The model under review builds one solid part; all positions refer to its coordinate system, in mm. Give positions to 0.01 mm unless a question says otherwise; leave off trailing zeros. Loops run counter-clockwise (first coordinate to the right, second up) from the corner with the lowest first, then second, coordinate; pieces in that order, holes last. Notation, with made-up numbers: (-29, 38) -> (-8, 38) arc R27 cw to (-8, 65) -> close; hole circle Ø11 at (49.5, 43). An arc over 180 degrees is marked (long way). Write each question's results on one line, items separated by ' | '. Start each with the question number.
Q1. We need section A-A (y = 0). Write out the cut boundary in (x, z) (3 decimals).
Q2. We need section B-B (x = 27). Write out the cut boundary in (y, z), plus the area to 3 significant figures.
Q3. Wall thickness on L1, parallel to X at y = 0, z = 0.45; L2, parallel to Y at x = 11.5, z = 0; L3, parallel to Y at x = 12.5, z = 0.8: over which ranges is each line inside the solid? List them lowest first. Write a range as [from, to].
Q4. Insertion check: pin 1 Ø1.4 at (x, y) = (26, 0) entering from -Z; pin 2 Ø2 at (y, z) = (-1.5, -1.5) entering from +X; pin 3 Ø1.5 at (x, z) = (13, 0.5) entering from +Y; pin 4 Ø3 at (y, z) = (0, 1) entering from -X. Each pin has a flat end and moves straight along its axis. Give the tip position at first contact, or say it passes through.
Q5. We need section C-C (x = 14.25). Write out the cut boundary in (y, z).
Q6. We need section D-D (x = 20). Write out the cut boundary in (y, z).
from build123d import *
from build123d.topology import SkipClean

# Parameters (mm, degrees)
BOSS_EXTRUDE1_DEPTH = 1
SKETCH5_R           = 0.9500000000000008
CUT_EXTRUDE1_DEPTH  = 2
FILLET1_R           = 0.3
SKETCH6_R           = 1
CUT_EXTRUDE2_DEPTH  = 15


with BuildPart() as part:
    # Sketch2 → Revolve1 (revolve)
    with BuildSketch(Plane.XY, mode=Mode.PRIVATE) as revolve1_sk:
        Polygon((0, 0), (0, 2.75), (4, 2.625), (4, 2.25), (24.5, 1.75), (24.5, 0), align=None)
    revolve(revolve1_sk.sketch.rotate(Axis((0, 0, 0), (1, 0, 0)), 90), axis=Axis((0, 0, 0), (1, 0, 0)))

    # Sketch3 → Boss-Extrude1 (add, symmetric)
    with BuildSketch(Plane.XY):
        with BuildLine():
            Line((24.5, 1.75), (24.5, -1.75))
            Line((24.5, -1.75), (27.61633950553443, -1.673991719377209))
            ThreePointArc((27.61633950553443, -1.673991719377209), (29.24999999999989, -1.262e-14), (27.61633950553443, 1.6739917193771834))
            Line((27.61633950553443, 1.6739917193771834), (24.5, 1.75))
        make_face()
    extrude(amount=BOSS_EXTRUDE1_DEPTH, both=True)

    # Sketch4 → Cut-Revolve1 (revolve, cut)
    with SkipClean():  # the faces are left unmerged after this step: merging them gives an invalid solid
        with BuildSketch(Plane.XY):
            Polygon((24.5, 1.75), (30.062821942046543, 1.6143214160476007), (30.062821942046543, 2.5), (24.5, 2.5), align=None)
        revolve(axis=Axis((24.5, 4.3e-16, 0), (1, -3e-16, 0)), mode=Mode.SUBTRACT)

    # Sketch5 → Cut-Extrude1 (cut)
    with SkipClean():  # the faces are left unmerged after this step: merging them gives an invalid solid
        with BuildSketch(Plane.XY.offset(1)):
            with Locations((27.575510439208156, -1.262e-14)):
                Circle(SKETCH5_R)
        extrude(amount=-CUT_EXTRUDE1_DEPTH, mode=Mode.SUBTRACT)

    # Fillet1
    fillet1_edges = [part.edges().sort_by_distance(p)[0] for p in [
        (28.132039020152703, 1.5793008628168437, -0.5158528825070366),
        (28.132039019923862, -1.579300862247398, -0.5158528822781783),
        (28.1320390201527, 1.579300862816838, 0.5158528825070365),
        (28.132039019899718, -1.5793008622559224, 0.5158528822537949),
    ]]
    fillet(fillet1_edges, radius=FILLET1_R)

    # Sketch6 → Cut-Extrude2 (cut)
    with SkipClean():  # the faces are left unmerged after this step: merging them gives an invalid solid
        with BuildSketch(Plane.ZY):
            Circle(SKETCH6_R)
        extrude(amount=-CUT_EXTRUDE2_DEPTH, mode=Mode.SUBTRACT)


solid = part.part
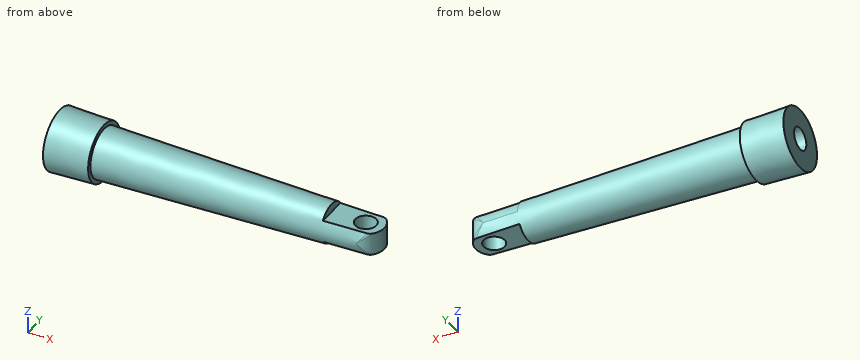
Output:
1) outline: (0, -2.75) -> (4, -2.625) -> (4, -2.25) -> (24.5, -1.75) -> (24.5, -1) -> (26.626, -1) -> (26.626, 1) -> (24.5, 1) -> (24.5, 1.75) -> (4, 2.25) -> (4, 2.625) -> (0, 2.75) -> (0, 1) -> (15, 1) -> (15, -1) -> (0, -1) -> close; (28.526, -1) -> (29.25, -1) -> (29.25, 1) -> (28.526, 1) -> close
2) outline: (-1.36, -1) -> (-0.76, -1) -> (-0.76, 1) -> (-1.36, 1) arc R1.69 ccw to start; (0.76, -1) -> (1.36, -1) arc R1.69 ccw to (1.36, 1) -> (0.76, 1) -> close | area: 3.31 mm2
3) L1: [15, 26.63], [28.53, 29.25] | L2: [-2.07, -1], [1, 2.07] | L3: [-1.88, -0.6], [0.6, 1.88]
4) pin 1: z = -1 | pin 2: x = 29.13 | pin 3: y = 2.04 | pin 4: x = 0
5) outline: circle Ø4 at (0, 0); hole circle Ø2 at (0, 0)
6) outline: circle Ø3.72 at (0, 0)
